Design review of the part built by this model. Coordinates are the model's own, in mm. A direction names the side the tool comes from. Give positions to 0.01 mm unless a question says otherwise; leave off trailing zeros. Loops run counter-clockwise (first coordinate to the right, second up) from the corner with the lowest first, then second, coordinate; pieces in that order, holes last. Notation, with made-up numbers: (63.25, 24.5) - (106.25, 24.5) arc R22 cw to (106.25, 37.5) - close; hole circle Ø10 at (-25, -27). An arc over 180 degrees is marked (long way). One line per item, written item: value. Start each with the question number.
```python
from build123d import *

# Parameters (mm, degrees)
SKETCH2_R           = 2.4
BOSS_EXTRUDE1_DEPTH = 11.2
SKETCH4_OUTSIDE_W   = 9.42
SKETCH4_OUTSIDE_H   = 9.42
SKETCH4_OUTSIDE_R   = 1.25
CUT_EXTRUDE1_DEPTH  = 9.3
SKETCH5_OUTSIDE_W   = 9.42
SKETCH5_OUTSIDE_H   = 9.42
SKETCH5_OUTSIDE_R   = 0.85
CUT_EXTRUDE2_DEPTH  = 3.4
SKETCH6_W           = 5
SKETCH6_H           = 0.6
CUT_EXTRUDE3_DEPTH  = 0.9
FILLET1_R           = 0.1
CHAMFER2_SIZE       = 0.2
CHAMFER1_SIZE       = 0.25


with BuildPart() as part:
    # Sketch2 → Boss-Extrude1 (new body)
    with BuildSketch(Plane.XY):
        Circle(SKETCH2_R)
    extrude(amount=-BOSS_EXTRUDE1_DEPTH)

    # Sketch4 outside → Cut-Extrude1 (cut)
    with BuildSketch(Plane(origin=(0, 0, -11.2), x_dir=(-1, 0, 0), z_dir=(0, 0, -1))):
        Rectangle(SKETCH4_OUTSIDE_W, SKETCH4_OUTSIDE_H)
        Circle(SKETCH4_OUTSIDE_R, mode=Mode.SUBTRACT)
    extrude(amount=-CUT_EXTRUDE1_DEPTH, mode=Mode.SUBTRACT)

    # Sketch5 outside → Cut-Extrude2 (cut)
    with BuildSketch(Plane(origin=(0, 0, -11.2), x_dir=(-1, 0, 0), z_dir=(0, 0, -1))):
        Rectangle(SKETCH5_OUTSIDE_W, SKETCH5_OUTSIDE_H)
        Circle(SKETCH5_OUTSIDE_R, mode=Mode.SUBTRACT)
    extrude(amount=-CUT_EXTRUDE2_DEPTH, mode=Mode.SUBTRACT)

    # Sketch6 → Cut-Extrude3 (cut)
    with BuildSketch(Plane.XY):
        Rectangle(SKETCH6_W, SKETCH6_H)
    extrude(amount=-CUT_EXTRUDE3_DEPTH, mode=Mode.SUBTRACT)

    # Fillet1
    fillet1_edges = [part.edges().sort_by_distance(p)[0] for p in [
        (1.25, 0, -1.9),
        (0.85, 0, -7.8),
    ]]
    fillet(fillet1_edges, radius=FILLET1_R)

    # Chamfer2
    chamfer2_edges = [part.edges().sort_by_distance(p)[0] for p in [
        (0, 2.4, 0),
        (0, -2.4, 0),
    ]]
    chamfer(chamfer2_edges, length=CHAMFER2_SIZE)

    # Chamfer1
    chamfer1_edges = [part.edges().sort_by_distance(p)[0] for p in [
        (0.85, 0, -11.2),
    ]]
    chamfer(chamfer1_edges, length=CHAMFER1_SIZE)


solid = part.part
```
(1) Take a section at D-D on z = -8.25. State the section outline as (x, y) points, and give its area (3 significant figures).
(2) Take a section at C-C on z = -1.75. State the section outline as (x, y) points.
(3) To check wall thickness, follow L1, parallel to Y at x = 0.05, z = -10.25; L2, parallel to Z at x = -1.3, y = 0.45; L3, parallel to Z at x = 0.7, y = 0.85. State the ranges of each line that lie inside material, in increasing order. Write a range as from..to.
(4) For pin 1 Ø1 at (x, z) = (-1, -0.5) entering from -Y; pin 2 Ø2 at (y, z) = (1, -5) entering from -X; pin 3 Ø1.4 at (x, y) = (0, -1) entering from -Z; pin 4 Ø1.5 at (x, y) = (-1.5, 0) entering from -Z, all flat-tipped, find the tip position at first contact; note any pin that passes through.
(5) Machinability: for faces 1 (the flat face through (0, -0.3, -0.4)), 2 (the flat face through (0, -2, -1.9)), 3 (the flat face through (0, 1, 0)), which of the approach directions +Z, -Z, +X, -X, +Y, -Y give a long, thin tool a straight path to every point of the face, cutting with its end or side? Answer none if there is none.
(6) Take a section at B-B on y = 0. State the section outline as (x, z) points, and give its area (3 significant figures).
(7) Draft analysis for pull direction Y (two halves, no side actions). For faces 4 (the cylindrical face through (2.29, 0.72, -1.04)), 5 (the flat face through (0, 0.3, -0.4)), 6 (the flat face through (0, 0, -11.2)), state which applies: pulls with the +Y half, pulls with the -Y half, needs draft (parallel to the pull), parting line crosses it, or undercut.
(8) Take a section at A-A on x = 0. State the section outline as (y, z) points.
Here are the results:
1. outline: circle Ø1.7 at (0, 0)
1. area: 2.27 mm²
2. outline: circle Ø4.8 at (0, 0)
3. L1: -0.85..0.85
3. L2: -1.9..0
3. L3: -7.8..0
4. pin 1: y = -2.35
4. pin 2: x = -1.25
4. pin 3: z = -11.2
4. pin 4: z = -11.05
5. face 1: +Z, +X, -X
5. face 2: -Z
5. face 3: +Z, +X, -X, +Y, -Y
6. outline: (-2.4, -1.9) - (-1.35, -1.9) arc R0.1 cw to (-1.25, -2) - (-1.25, -7.8) - (-0.95, -7.8) arc R0.1 cw to (-0.85, -7.9) - (-0.85, -10.95) - (-0.6, -11.2) - (0.6, -11.2) - (0.85, -10.95) - (0.85, -7.9) arc R0.1 cw to (0.95, -7.8) - (1.25, -7.8) - (1.25, -2) arc R0.1 cw to (1.35, -1.9) - (2.4, -1.9) - (2.4, -0.9) - (-2.4, -0.9) - close
6. area: 25.3 mm²
7. face 4: parting line crosses it
7. face 5: undercut
7. face 6: needs draft
8. outline: (-2.4, -1.9) - (-1.35, -1.9) arc R0.1 cw to (-1.25, -2) - (-1.25, -7.8) - (-0.95, -7.8) arc R0.1 cw to (-0.85, -7.9) - (-0.85, -10.95) - (-0.6, -11.2) - (0.6, -11.2) - (0.85, -10.95) - (0.85, -7.9) arc R0.1 cw to (0.95, -7.8) - (1.25, -7.8) - (1.25, -2) arc R0.1 cw to (1.35, -1.9) - (2.4, -1.9) - (2.4, -0.2) - (2.2, 0) - (0.3, 0) - (0.3, -0.9) - (-0.3, -0.9) - (-0.3, 0) - (-2.2, 0) - (-2.4, -0.2) - close
